Could you check a few things on this model? Use its own coordinates, in mm. A direction names the side the tool comes from. Give positions to 0.01 mm unless a question says otherwise; leave off trailing zeros. Order: outer loops, then holes, each group sorted by start corner. A loop starts at its lowest first (then second) coordinate and runs counter-clockwise, first axis right, second up. Notation, with made-up numbers: (30, 31.25) - (88, 31.25) arc R7 cw to (88, 39.25) - close; hole circle Ø6 at (57, 74.5). An arc over 180 degrees is marked (long way). Put each result on its own line as item: value.
Autodesk Inventor part; units mm, degrees
ref_plane "YZ Plane" through (0, 0, 0) normal (1, 0, 0) x (0, 1, 0)
ref_plane "XZ Plane" through (0, 0, 0) normal (0, 1, 0) x (-1, 0, 0)
ref_plane "XY Plane" through (0, 0, 0) normal (0, 0, 1) x (1, 0, 0)
sketch "Sketch1" plane through (0, 0, 0) normal (0, 0, 1) x (1, 0, 0)
  circle A0 centre (0, 0) radius 3.175
  dimension "d0" = 6.35
extrude "Extrusion1" add sketch "Sketch1" along normal blind 19.05
sketch "Sketch2" plane through (0, 0, 0) normal (0, 0, -1) x (-1, 0, 0)
  circle A0 centre (0, 0) radius 3.175
  circle A1 centre (0, 0) radius 4.7625
  dimension "d3" = 9.525
extrude "Extrusion2" add sketch "Sketch2" along normal blind 6.35 contours A0 | A1
sketch "Sketch3" plane through (0, 0, -6.35) normal (0, 0, -1) x (-1, 0, 0)
  circle A0 centre (0, 0) radius 4.7625
  line L0 (-1.3748, 2.3812) -> (1.3748, 2.3813)
  line L1 (1.3748, 2.3813) -> (2.7496, 0)
  line L2 (2.7496, 0) -> (1.3748, -2.3812)
  line L3 (1.3748, -2.3812) -> (-1.3748, -2.3812)
  line L4 (-1.3748, -2.3812) -> (-2.7496, 0)
  line L5 (-2.7496, 0) -> (-1.3748, 2.3812)
  dimension "d6" = 4.7625
extrude "Extrusion3" cut sketch "Sketch3" against normal blind 3.175 contours L0 L1 L2 L3 L4 L5
chamfer "Chamfer1" distance 0.508 angle 45 3 edges at (-3.175, 0, 19.05) (4.7625, 0, 0) (4.7625, 0, -6.35)
thread "Thread1"
properties part number "14-20 x750" material "Steel"
1) Suppose I cut it at C-C, the plane z = 15.5. List the corners of the cut face in (x, y) for me (3 decimals).
Filled in:
outline: circle Ø6.35 at (0, 0)
2) I'm going to push flat-ended pins straight in: pin 1 (1.5 mm diameter, centred on x = 3.5, z = -2.5, fed in from +Y); pin 2 (1.5 mm diameter, centred on y = 1.5, z = 15, fed in from +X); pin 3 (1 mm diameter, centred on x = 2, z = -0.5, fed in from -Y). Where does each tip first touch, or does it pass through?
Filled in:
pin 1: stops at y = 3.89
pin 2: stops at x = 3.09
pin 3: stops at y = -4.52
3) If I drill on line 1 (Z direction, x = 2, y = -3.75); line 2 (Z direction, x = 0.25, y = -0.5) (3 decimals); line 3 (Y direction, x = -2, z = -3.25), over which ranges is the centre line in solid material (lowest first)? Write a range as [from, to].
Filled in:
line 1: z = [-6.35, 0]
line 2: z = [-3.175, 19.05]
line 3: y = [-4.32, -1.3], [1.3, 4.32]
4) Which directions (+Z, -Z, +X, -X, +Y, -Y) give clear straight access to the entire face, cutting with the end or side of a thin tool? Please do faces 1 (the flat face through (2.05, -1.21, -4.78)), 2 (the flat face through (2, -3, 0)), 3 (the flat face through (0, 0, 19.05)).
Filled in:
face 1: -Z
face 2: +Z
face 3: +Z, +X, -X, +Y, -Y
5) Suppose I cut it at A-A, the plane z = -1. List the corners of the cut face in (x, y) for me (1 decimal).
Filled in:
outline: circle Ø9.5 at (0, 0)
6) We'd pull the mould along X, two halves only. Please class faces 4 (the cylindrical face through (-0.69, 3.1, 9.14)), 5 (the flat face through (-2, -2, -6.35)), 6 (the flat face through (2.072, 1.174, -4.785)): pulls with the +X half, pulls with the -X half, needs draft (parallel to the pull), parting line crosses it, or undercut.
Filled in:
face 4: parting line crosses it
face 5: needs draft
face 6: undercut
